CAD build for the part. Positions are in the model's coordinates, mm. A direction names the side the tool comes from. Give positions to 0.01 mm unless a question says otherwise; leave off trailing zeros. Order: outer loops, then holes, each group sorted by start corner. A loop starts at its lowest first (then second) coordinate and runs counter-clockwise, first axis right, second up. Notation, with made-up numbers: (62.5, -20) -> (100.5, -20) arc R21 cw to (100.5, -7) -> close; hole circle Ø10 at (30, 61). An arc over 180 degrees is marked (long way). Use one line per item in the form item = value. Start each with the question number.
1) Tool access for faces 1 (the face through (-45, -1, 2)), 2 (the face through (0, -12, 2)): list every direction of +Z, -Z, +X, -X, +Y, -Y with a clear straight run to the whole face (end or side of a thin tool).
2) Cut at B-B, the plane z = 3.25. Give the cut face in (x, y), and give its area (3 significant figures).
3) Cut at C-C, the plane y = -22. Give the cut face in (x, z), and give its area (3 significant figures).
4) Drop a flat-ended pin along its axis: P1, Ø4.5, axis at x = 36, y = -48, coming from the +Z side. Give the stop position or say it passes through.
5) Cut at D-D, the plane x = -36. Give the cut face in (y, z), and give its area (3 significant figures).
6) Probe line 1 (Y direction, x = -36, z = 1.15); line 2 (Y direction, x = -23, z = 2.9); line 3 (X direction, y = -17.5, z = 2.2). List the from-to ranges inside material, lowest first.
7) Cut at A-A, the plane x = 29. Give the cut face in (y, z).
8) Mould opens along Y. For faces 3 (the face through (-1, 82, 2)), 4 (the face through (-1, -17, 4)), 5 (the face through (-28.5, -16.9, 2)), 6 (the face through (-12, 25, 2)) say: pulls with the +Y half, pulls with the -Y half, needs draft (parallel to the pull), parting line crosses it, or undercut.
from build123d import *

# Parameters (mm, degrees)
SKETCH_1_W      = 90
SKETCH_1_H      = 164
SKETCH_1_R      = 2
SKETCH_1_R_2    = 7.5
EXTRUDE_1_DEPTH = 4


with BuildPart() as part:
    # 草图1 → 凸台-拉伸1 (new body)
    with BuildSketch(Plane.XY):
        Rectangle(SKETCH_1_W, SKETCH_1_H)
        with Locations((-36, 48)):
            Circle(SKETCH_1_R, mode=Mode.SUBTRACT)
        with Locations((-36, -48)):
            Circle(SKETCH_1_R, mode=Mode.SUBTRACT)
        with Locations(Location((36, -48, 0), (0, 0, 180))):
            Circle(SKETCH_1_R, mode=Mode.SUBTRACT)
        with Locations(Location((36, 48, 0), (0, 0, 180))):
            Circle(SKETCH_1_R, mode=Mode.SUBTRACT)
        with Locations((-23, -22)):
            Circle(SKETCH_1_R_2, mode=Mode.SUBTRACT)
        with Locations(Location((23, -22, 0), (0, 0, 180))):
            Circle(SKETCH_1_R_2, mode=Mode.SUBTRACT)
        with BuildLine():
            Line((-12, 0), (-12, 50))
            ThreePointArc((-12, 50), (0, 62), (12, 50))
            Line((12, 50), (12, 0))
            ThreePointArc((12, 0), (0, -12), (-12, 0))
        make_face(mode=Mode.SUBTRACT)
    extrude(amount=EXTRUDE_1_DEPTH)


solid = part.part
Result:
q1.face_1 = +Z, -Z, -X, +Y, -Y
q1.face_2 = +Z, -Z
q2.outline = (-45, -82) -> (45, -82) -> (45, 82) -> (-45, 82) -> close; hole circle Ø4 at (-36, -48); hole circle Ø4 at (-36, 48); hole circle Ø15 at (-23, -22); hole (-12, 0) arc R12 ccw to (12, 0) -> (12, 50) arc R12 ccw to (-12, 50) -> close; hole circle Ø15 at (23, -22); hole circle Ø4 at (36, -48); hole circle Ø4 at (36, 48)
q2.area = 12,700 mm²
q3.outline = (-45, 0) -> (-30.5, 0) -> (-30.5, 4) -> (-45, 4) -> close; (-15.5, 0) -> (15.5, 0) -> (15.5, 4) -> (-15.5, 4) -> close; (30.5, 0) -> (45, 0) -> (45, 4) -> (30.5, 4) -> close
q3.area = 240 mm²
q4.P1 = 4
q5.outline = (-82, 0) -> (-50, 0) -> (-50, 4) -> (-82, 4) -> close; (-46, 0) -> (46, 0) -> (46, 4) -> (-46, 4) -> close; (50, 0) -> (82, 0) -> (82, 4) -> (50, 4) -> close
q5.area = 624 mm²
q6.line_1 = -82 to -50, -46 to 46, 50 to 82
q6.line_2 = -82 to -29.5, -14.5 to 82
q6.line_3 = -45 to -29, -17 to 17, 29 to 45
q7.outline = (-82, 0) -> (-26.5, 0) -> (-26.5, 4) -> (-82, 4) -> close; (-17.5, 0) -> (82, 0) -> (82, 4) -> (-17.5, 4) -> close
q8.face_3 = pulls with the +Y half
q8.face_4 = needs draft
q8.face_5 = undercut
q8.face_6 = undercut
